```python
from build123d import *

# Parameters (mm, degrees)
F0_W     = 6.35
F0_H     = 31.75
F0_R     = 1.6764
F1_DEPTH = 3.175
F2_SIZE  = 0.254


with BuildPart() as f1:
    # F0 (on Front) → F1 (new body)
    with BuildSketch(Plane.XZ):
        Rectangle(F0_W, F0_H)
        with Locations((0, -9.525)):
            Circle(F0_R, mode=Mode.SUBTRACT)
        with Locations((0, 3.175)):
            Circle(F0_R, mode=Mode.SUBTRACT)
    extrude(amount=F1_DEPTH)

    # F2
    f2_edges = [f1.edges().sort_by_distance(p)[0] for p in [
        (-1.6764, -3.175, 3.175),
        (-1.6764, -3.175, -9.525),
        (3.175, -1.5875, -15.875),
        (-3.175, -1.5875, 15.875),
        (3.175, -1.5875, 15.875),
        (-1.6764, 0, -9.525),
        (-3.175, -1.5875, -15.875),
        (0, 0, -15.875),
        (0, -3.175, -15.875),
        (0, 0, 15.875),
        (0, -3.175, 15.875),
        (-3.175, 0, 0),
        (-3.175, -3.175, 0),
        (3.175, 0, 0),
        (3.175, -3.175, 0),
        (-1.6764, 0, 3.175),
    ]]
    chamfer(f2_edges, length=F2_SIZE)


solid = f1.part
```
Geometry check sheet. Reference: the model listing, model coordinates, mm. Coordinates: 2 decimals unless noted, no trailing zeros. Loops run counter-clockwise (first coordinate to the right, second up) from the corner with the lowest first, then second, coordinate; pieces in that order, holes last.
Item 1: Thickness scan on line 1 (Z direction, x = 0, y = -1.95) (3 decimals); line 2 (Z direction, x = 0.25, y = -0.9) (3 decimals); line 3 (X direction, y = -1.3, z = -10.5) (3 decimals). Record the ranges inside material, lowest first.
Item 2: Sectioned sample at B-B, the plane y = -1.3. Record the boundary of the cut face in (x, z) (3 decimals).
Item 3: Release check for a two-part mould opening along Z. For faces 1 (the face through (0, -2, -15.875)), 2 (the face through (0.8, -1.6, -11)), 3 (the face through (3.175, -2, 0)) record: released by +Z, released by -Z, zero draft, split by the parting line, or undercut.
Item 4: Sectioned sample at A-A, the plane x = 0. Record the boundary of the cut face in (y, z) (3 decimals).
Check result:
1. line 1: z = -15.875 to -11.201, -7.849 to 1.499, 4.851 to 15.875
1. line 2: z = -15.875 to -11.183, -7.867 to 1.517, 4.833 to 15.875
1. line 3: x = -3.175 to -1.364, 1.364 to 3.175
2. outline: (-3.175, -15.621) - (-2.921, -15.875) - (2.921, -15.875) - (3.175, -15.621) - (3.175, 15.621) - (2.921, 15.875) - (-2.921, 15.875) - (-3.175, 15.621) - close; hole circle Ø3.353 at (0, -9.525); hole circle Ø3.353 at (0, 3.175)
3. face 1: released by -Z
3. face 2: undercut
3. face 3: zero draft
4. outline: (-3.175, -15.621) - (-2.921, -15.875) - (-0.254, -15.875) - (0, -15.621) - (0, -11.455) - (-0.254, -11.201) - (-2.921, -11.201) - (-3.175, -11.455) - close; (-3.175, -7.595) - (-2.921, -7.849) - (-0.254, -7.849) - (0, -7.595) - (0, 1.245) - (-0.254, 1.499) - (-2.921, 1.499) - (-3.175, 1.245) - close; (-3.175, 5.105) - (-2.921, 4.851) - (-0.254, 4.851) - (0, 5.105) - (0, 15.621) - (-0.254, 15.875) - (-2.921, 15.875) - (-3.175, 15.621) - close
